Part print with two shaded views. Sizes in mm from the minimum x, y, z corner. Give positions to 0.01 mm unless a question says otherwise; leave off trailing zeros. Loops run counter-clockwise (first coordinate to the right, second up) from the corner with the lowest first, then second, coordinate; pieces in that order, holes last. Notation, with made-up numbers: M 28.25,-10 L 78.25,-10 A16 cw 78.25,10 Z; hole C 27.5,-33.75 d9. An arc over 180 degrees is marked long. Answer in a Markdown table with one row per item.
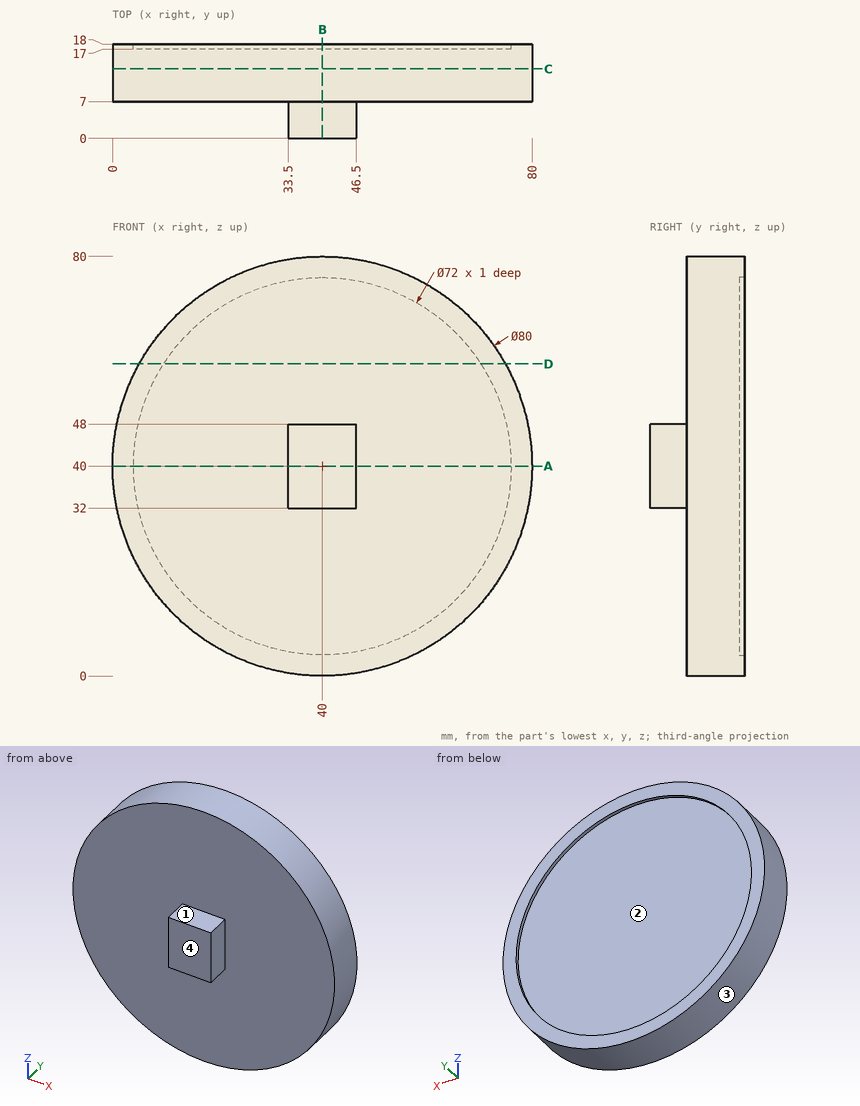
Q1. Saw through at D-D (z = 59.5). Give the cut face in (x, y).
Reported:
| item | result |
|---|---|
| outline | M 5.08,7 L 74.92,7 L 74.92,18 L 70.26,18 L 70.26,17 L 9.74,17 L 9.74,18 L 5.08,18 Z |
Q2. Drop flat-ended pins along their axis: pin 1 (3 mm diameter, centred on y = 10, z = 17, fed in from +X); pin 2 (4 mm diameter, centred on x = 19.5, y = 15.5, fed in from -Z); pin 3 (4 mm diameter, centred on x = 38, y = 6, fed in from +Z). Give the stop position or say it passes through.
Reported:
| item | result |
|---|---|
| pin 1 | x = 73.73 |
| pin 2 | z = 4.54 |
| pin 3 | z = 80 |
Q3. Saw through at B-B (x = 40). Give the cut face in (y, z).
Reported:
| item | result |
|---|---|
| outline | M 0,32 L 7,32 L 7,0 L 18,0 L 18,4 L 17,4 L 17,76 L 18,76 L 18,80 L 7,80 L 7,48 L 0,48 Z |
Q4. Probe probe 1 along X at (y, z) = (17.65, 40); probe 2 along Y at (x, z) = (65.5, 41.5); probe 3 along Y at (x, z) = (4.5, 54.5). List the from-to ranges inside material, lowest first.
Reported:
| item | result |
|---|---|
| probe 1 | 0 to 4, 76 to 80 |
| probe 2 | 7 to 17 |
| probe 3 | 7 to 18 |
Q5. Mould opens along Z. For the marked faces 1, 2, 3 and 4 say: released by +Z, released by -Z, zero draft, split by the parting line, or undercut.
Reported:
| item | result |
|---|---|
| face 1 | released by +Z |
| face 2 | undercut |
| face 3 | split by the parting line |
| face 4 | zero draft |
Q6. Saw through at A-A (z = 40). Give the cut face in (x, y), and give its area (3 significant figures).
Reported:
| item | result |
|---|---|
| outline | M 0,7 L 33.5,7 L 33.5,0 L 46.5,0 L 46.5,7 L 80,7 L 80,18 L 76,18 L 76,17 L 4,17 L 4,18 L 0,18 Z |
| area | 899 mm² |
Q7. Saw through at C-C (y = 13.25). Give the cut face in (x, z), and give its area (3 significant figures).
Reported:
| item | result |
|---|---|
| outline | C 40,40 d80 |
| area | 5,030 mm² |
